```python
from build123d import *

# Parameters (mm, degrees)
MAIN_BODY_DEPTH      = 18
SKETCH14_W           = 4.2
SKETCH14_H           = 39
M8_CLEARANCE_HOLE2_D = 8.4
M8_CLEARANCE_HOLE3_D = 8.4
SKETCH27_R           = 7
CUT_EXTRUDE2_DEPTH   = 99.559772913


with BuildPart() as part:
    # Sketch1 → main body (new body)
    with BuildSketch(Plane.XY):
        with BuildLine():
            Line((0, -48.600411521), (0, -83.600411521))
            Line((0, -83.600411521), (-10, -83.600411521))
            Line((-10, -83.600411521), (-10, -48.600411521))
            add(Edge.make_bspline(
                [(-26.535230031, -29.931280748), (-20.948212629, -34.88438627), (-10, -40.904022772), (-10, -48.600411521)],
                knots=[0, 0, 0, 0, 1, 1, 1, 1], degree=3))
            ThreePointArc((-26.535230031, -29.931280748), (-39.998128482, 0.386934068), (-25.951219512, 30.43902439))
            ThreePointArc((-25.951219512, 30.43902439), (-18.607817439, 40.126684972), (-16, 52))
            Line((-16, 52), (-1, 52))
            Line((-1, 52), (-1, 29.983328701))
            ThreePointArc((-1, 29.983328701), (0, -30), (1, 29.983328701))
            Line((1, 29.983328701), (1, 52))
            Line((1, 52), (9, 52))
            ThreePointArc((9, 52), (11.695932832, 42.212959957), (19.02319236, 35.186903138))
            ThreePointArc((19.02319236, 35.186903138), (39.54457484, -6.018853774), (7.693084301, -39.253234949))
            ThreePointArc((7.693084301, -39.253234949), (2.170592409, -42.547452411), (0, -48.600411521))
        make_face()
    extrude(amount=MAIN_BODY_DEPTH)

    # Sketch14 → M8 Clearance Hole1 (revolve, cut)
    with BuildSketch(Plane(origin=(1, 43, 9), x_dir=(0, 0, 1), z_dir=(0, 1, 0))):
        with Locations((2.1, 19.5)):
            Rectangle(SKETCH14_W, SKETCH14_H)
    revolve(axis=Axis((-5.35, 43, 9), (1, 0, 0)), mode=Mode.SUBTRACT)

    # M8 Clearance Hole2 (through all)
    with Locations(Plane(origin=(1, 0, 0), x_dir=(0, 0, 1), z_dir=(1, 0, 0))):
        with Locations((9, -43)):
            Hole(M8_CLEARANCE_HOLE2_D / 2)

    # M8 Clearance Hole3 (through all)
    with Locations(Plane(origin=(0, 0, 0), x_dir=(0, 0, -1), z_dir=(1, 0, 0))):
        with Locations((-9, -55.600411521), (-9, -73.100411521)):
            Hole(M8_CLEARANCE_HOLE3_D / 2)

    # Sketch27 → Cut-Extrude2 (cut, through all)
    with BuildSketch(Plane(origin=(9, 0, 0), x_dir=(0, 0, -1), z_dir=(1, 0, 0))):
        with Locations(Location((-9, 43, 0), (0, 0, 270))):
            Circle(SKETCH27_R)
    extrude(amount=CUT_EXTRUDE2_DEPTH, mode=Mode.SUBTRACT)


solid = part.part
```
The listing builds one solid part. Answer for the finished solid, in the listing's coordinates (mm). A direction names the side the tool comes from. Coordinates: 2 decimals unless noted, no trailing zeros. Loops run counter-clockwise (first coordinate to the right, second up) from the corner with the lowest first, then second, coordinate; pieces in that order, holes last. Notation, with made-up numbers: (-33, 34) - (1, 34) arc R23 ccw to (1, 47) - close; hole circle Ø11 at (77, -4). An arc over 180 degrees is marked (long way). Use a Markdown table: item, result. Add a question column.
1) For faces 1 (the cylindrical face through (5.056, 38.836, 8.453)), 2 (the flat face through (-10, -66, 9)), 3 (the flat face through (1, 38, 9)), determine the directions among +Z, -Z, +X, -X, +Y, -Y from which every point of the face is accessible in a straight line to the end or side of a thin tool.
2) The part is cut by section B-B, the plane y = 43. Give the vertices of the cut face in (x, z), and give its area (3 significant figures).
3) The part is cut by section C-C, the plane x = -12.5. State how many separate pieces and enclosed holes the cut face has, and give its area (3 significant figures).
4) Given pin 1 (4 mm diameter, centred on y = -59.5, z = 6, fed in from -X); pin 2 (9 mm diameter, centred on y = -69, z = 13, fed in from +X); pin 3 (2 mm diameter, centred on x = -29, z = 14, fed in from -Y); pin 4 (2 mm diameter, centred on x = -3, y = 30, fed in from -Z), each flat-ended and moving along its own axis, determine where each tip first touches the part or whether it passes through.
5) The mould has two halves that part along Y. Classify faces 4 (the flat face through (0, -66, 9)), 5 (the cylindrical face through (12.306, 36.323, 6.897)), 6 (the flat face through (9, 43, 14)), 7 (the cylindrical face through (-19.95, 37.57, 8.87)): released by +Y, released by -Y, zero draft, split by the parting line, or undercut.
6) Find the intervals of material crossed by line 1 (Z direction, x = -12, y = 43); line 2 (Y direction, x = -4.5, z = 9); line 3 (Y direction, x = 3.75, z = 9), in increasing order.
7) The part is cut by section A-A, the plane y = 0. Give the vertices of the cut face in (x, z).
Here are the results:
| question | item | result |
|---|---|---|
| 1 | face 1 | +X, -X |
| 1 | face 2 | +Z, -Z, -X, -Y |
| 1 | face 3 | +Z, -Z, +Y |
| 2 | outline | (-17.47, 0) - (-1, 0) - (-1, 4.8) - (-17.47, 4.8) - close; (-17.47, 13.2) - (-1, 13.2) - (-1, 18) - (-17.47, 18) - close; (1, 0) - (11.25, 0) - (11.25, 2) - (9, 2) - (9, 4.8) - (1, 4.8) - close; (1, 13.2) - (9, 13.2) - (9, 16) - (11.25, 16) - (11.25, 18) - (1, 18) - close |
| 2 | area | 244 mm^2 |
| 3 | separate pieces | 2 |
| 3 | enclosed holes | 1 |
| 3 | area | 657 mm^2 |
| 4 | pin 1 | stops at x = -10 |
| 4 | pin 2 | stops at x = 0 |
| 4 | pin 3 | stops at y = -28.57 |
| 4 | pin 4 | stops at z = 0 |
| 5 | face 4 | zero draft |
| 5 | face 5 | undercut |
| 5 | face 6 | undercut |
| 5 | face 7 | released by +Y |
| 6 | line 1 | z = 0 to 4.8, 13.2 to 18 |
| 6 | line 2 | y = -83.6 to -77.3, -68.9 to -59.8, -51.4 to -29.66, 29.66 to 38.8, 47.2 to 52 |
| 6 | line 3 | y = -41.03 to -29.76, 29.76 to 38.8, 47.2 to 52 |
| 7 | outline | (-40, 0) - (-30, 0) - (-30, 18) - (-40, 18) - close; (30, 0) - (40, 0) - (40, 18) - (30, 18) - close |
